Geometry: see drawing. Coordinates: mm, zero at the bounding-box minimum. Round coordinates to 2 decimals unless told otherwise and drop trailing zeros. Loops run counter-clockwise (first coordinate to the right, second up) from the corner with the lowest first, then second, coordinate; pieces in that order, holes last. Notation, with made-up numbers: (69, -10) - (112, -10) arc R25 cw to (112, 29) - close; hole circle Ø4 at (-32.5, 52). An arc over 180 degrees is marked (long way). Write item = value, one per line. Start each with the question number.
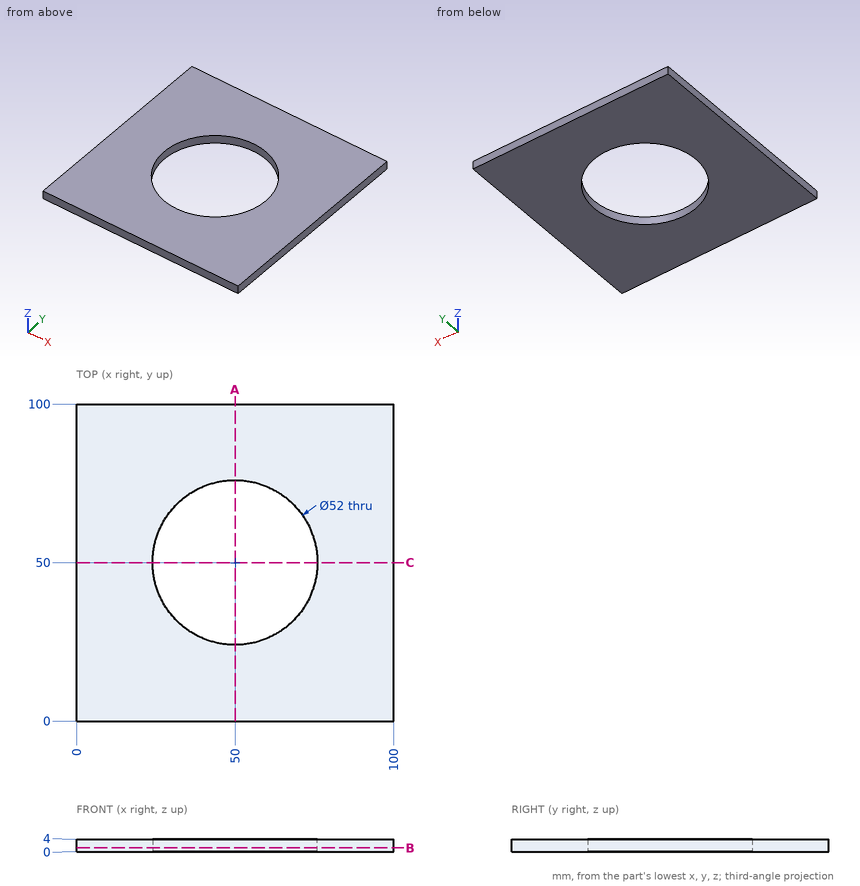
(1) Material intervals for line 1 along X through (y, z) = (50, 2.7); line 2 along X through (y, z) = (28.5, 3.6), sorted ascending. Write a range as from..to.
(2) Cut plane A-A (x = 50). Output: boundary loops of the cut face in (y, z).
(3) Cut plane B-B (z = 1.2). Output: boundary loops of the cut face in (x, y).
Solution:
q1.line_1 = 0..24, 76..100
q1.line_2 = 0..35.38, 64.62..100
q2.outline = (0, 0) - (24, 0) - (24, 4) - (0, 4) - close; (76, 0) - (100, 0) - (100, 4) - (76, 4) - close
q3.outline = (0, 0) - (100, 0) - (100, 100) - (0, 100) - close; hole circle Ø52 at (50, 50)
